Geometry: final body of the model. Coordinates: model frame, mm. Face numbers are marked on the shaded views. A direction names the side the tool comes from. Round coordinates to 2 decimals unless told otherwise and drop trailing zeros. Loops run counter-clockwise (first coordinate to the right, second up) from the corner with the lowest first, then second, coordinate; pieces in that order, holes last. Notation, with made-up numbers: (8, -23) - (55, -23) arc R19 cw to (55, 3) - close; hole circle Ø6 at (-24.5, -0.75). An arc over 180 degrees is marked (long way). Return JSON: item names as keys, results as strings. Group by question number.
1. Section A-A on z = 0. Return loops of the section in (x, y), and give its area (3 significant figures).
2. First-contact query: pin 1 Ø6 at (x, z) = (8, 6) entering from +Y. Flat tip, straight axial feed; report the tip coordinate or a pass-through.
3. Material intervals for probe 1 along X at (y, z) = (0.2, 0); probe 2 along Y at (x, z) = (18, 3); probe 3 along X at (y, z) = (-0.45, 10), sorted ascending.
4. Draft query along Z for the marked faces 3 and 4. Return one class per face: +Z half, -Z half, draft (parallel to the pull), parting line (faces both ways), or undercut.
5. Section C-C on y = 0.7. Return loops of the section in (x, z), and give its area (3 significant figures).
6. Set-up query: the marked faces 1 and 2. Return all of +Z, -Z, +X, -X, +Y, -Y with unobstructed straight access to the full face (end or side cutting, diameter ignored); none if empty.
7. Section B-B on x = 0. Return loops of the section in (y, z).
from build123d import *

# Parameters (mm, degrees)
CONG_1_R = 0.7
CONG_2_R = 0.2


with BuildPart() as part:
    # Esquisse1 → Base-Révol.-Mince (revolve)
    with BuildSketch(Plane.XY, mode=Mode.PRIVATE) as base_r_vol_mince_sk:
        Polygon((-26, 1), (-20, 1), (-20, 0), (-15, 0), (-15, -1), (-21, -1), (-21, 0), (-26, 0), align=None)
    revolve(base_r_vol_mince_sk.sketch.rotate(Axis((0, 0, 0), (0, -1, 0)), 90), axis=Axis((0, 0, 0), (0, -1, 0)))

    # Congé1
    cong_1_edges = [part.edges().sort_by_distance(p)[0] for p in [
        (0, 1, 20),
        (0, -1, 21),
    ]]
    fillet(cong_1_edges, radius=CONG_1_R)

    # Congé2
    cong_2_edges = [part.edges().sort_by_distance(p)[0] for p in [
        (0, 0, 20),
    ]]
    fillet(cong_2_edges, radius=CONG_2_R)


solid = part.part
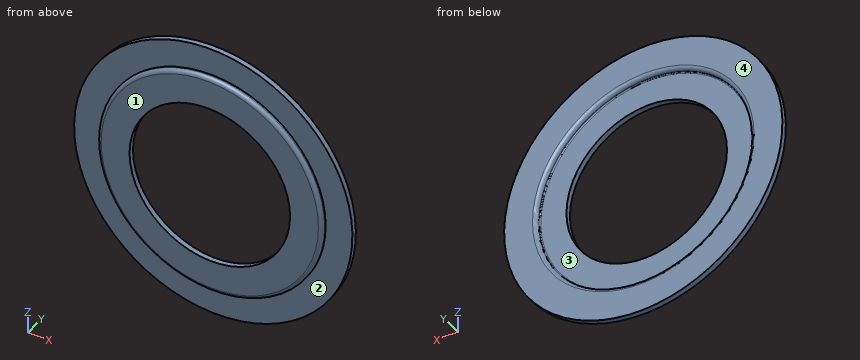
Taken from the geometry:
{
 "1": {"outline": "(-26, 0) - (-21, 0) - (-21, -0.3) arc R0.7 ccw to (-20.3, -1) - (-15, -1) - (-15, 0) - (-19.8, 0) arc R0.2 cw to (-20, 0.2) - (-20, 0.3) arc R0.7 ccw to (-20.7, 1) - (-26, 1) - close; (15, -1) - (20.3, -1) arc R0.7 ccw to (21, -0.3) - (21, 0) - (26, 0) - (26, 1) - (20.7, 1) arc R0.7 ccw to (20, 0.3) - (20, 0.2) arc R0.2 cw to (19.8, 0) - (15, 0) - close", "area": "23.6 mm2"},
 "2": {"pin 1": "through"},
 "3": {"probe 1": "-26 to -20, 20 to 26", "probe 2": "-1 to 0", "probe 3": "-18.45 to -11.18, 11.18 to 18.45"},
 "4": {"face 3": "undercut", "face 4": "draft"},
 "5": {"outline": "circle Ø52 at (0, 0); hole circle Ø40.25 at (0, 0)", "area": "851 mm2"},
 "6": {"face 1": "+Z, -Z, +X, -X, -Y", "face 2": "-Y"},
 "7": {"outline": "(-1, -20.3) arc R0.7 ccw to (-0.3, -21) - (0, -21) - (0, -26) - (1, -26) - (1, -20.7) arc R0.7 ccw to (0.3, -20) - (0.2, -20) arc R0.2 cw to (0, -19.8) - (0, -15) - (-1, -15) - close; (-1, 15) - (0, 15) - (0, 19.8) arc R0.2 cw to (0.2, 20) - (0.3, 20) arc R0.7 ccw to (1, 20.7) - (1, 26) - (0, 26) - (0, 21) - (-0.3, 21) arc R0.7 ccw to (-1, 20.3) - close"}
}
